Design review of the part built by this model. Coordinates are the model's own, in mm. A direction names the side the tool comes from. Give positions to 0.01 mm unless a question says otherwise; leave off trailing zeros. Write each loop counter-clockwise with the first axis right and the second up, starting at its lowest first coordinate (ties: lowest second). Pieces come first, ordered by that corner, then holes.
```python
from build123d import *

# Parameters (mm, degrees)
BOSS_EXTRUDE1_DEPTH = 304.8
SKETCH4_R           = 6.35
CUT_EXTRUDE1_DEPTH  = 599.68125614
SKETCH5_W           = 541.53125614
SKETCH5_H           = 3.114661147
BOSS_EXTRUDE2_DEPTH = 152.4


with BuildPart() as part:
    # Sketch1 → Boss-Extrude1 (new body)
    with BuildSketch(Plane(origin=(0, 0, 0), x_dir=(1, 0, 0), z_dir=(0, 1, 0))):
        Polygon((595.50625614, 4.567872613), (3.175, 4.567872613), (3.175, -53.975), (0, -53.975), (0, 0), (0, 7.742872613), (598.68125614, 7.742872613), (598.68125614, 4.567872613), (598.68125614, -49.407127387), (595.50625614, -49.407127387), align=None)
    extrude(amount=BOSS_EXTRUDE1_DEPTH)

    # Sketch4 → Cut-Extrude1 (cut, through all)
    with BuildSketch(Plane.ZY):
        with Locations((23.116063694, 152.4)):
            Circle(SKETCH4_R)
    extrude(amount=-CUT_EXTRUDE1_DEPTH, mode=Mode.SUBTRACT)

    # Sketch5 → Boss-Extrude2 (add)
    with BuildSketch(Plane(origin=(0, 304.8, 0), x_dir=(1, 0, 0), z_dir=(0, 1, 0))):
        with Locations((299.34062807, 6.088586102)):
            Rectangle(SKETCH5_W, SKETCH5_H)
    extrude(amount=BOSS_EXTRUDE2_DEPTH)


solid = part.part
```
(1) Consider section B-B, the plane z = 43. Give the boundary of the cut face in (x, y) (3 decimals).
Resolved:
outline: (0, 0) - (3.175, 0) - (3.175, 304.8) - (0, 304.8) - close; (595.506, 0) - (598.681, 0) - (598.681, 304.8) - (595.506, 304.8) - close
(2) Tool access review of faces 1 (the face through (301, 0, -7)), 2 (the face through (595.506, 150, 17)): name each direction out of +Z, -Z, +X, -X, +Y, -Y from which nothing blocks a thin tool from reaching the whole face with its end or side.
Resolved:
face 1: +Z, -Z, +X, -X, -Y
face 2: +Z, +Y, -Y
(3) Consider section D-D, the plane y = 323. Give the boundary of the cut face in (x, z) (3 decimals).
Resolved:
outline: (28.575, -7.646) - (570.106, -7.646) - (570.106, -4.531) - (28.575, -4.531) - close
(4) To check wall thickness, follow L1, parallel to X at y = 199, z = 3 (3 decimals); L2, parallel to Z at x = 1, y = 152 (3 decimals); L3, parallel to Z at x = 548, y = 109. State the ranges of each line that lie inside material, in increasing order.
Resolved:
L1: x = 0 to 3.175, 595.506 to 598.681
L2: z = -7.743 to 16.779, 29.453 to 53.975
L3: z = -7.74 to -4.57
(5) Clearance check with flat-ended pins moving along their axes: P1, Ø10, axis at x = 200, y = 339, coming from the +Z side; P2, Ø3, axis at x = 233.5, y = 206, coming from the +Z side; P3, Ø1.6, axis at y = 345, z = -6, coming from the -X side (3 decimals). State where each tip first meets the part, or that it passes through.
Resolved:
P1: stops at z = -4.53
P2: stops at z = -4.57
P3: stops at x = 28.575
(6) Mouldability with a two-part tool opening along Z and no side actions: class faces 3 (the face through (303, 150, -4.568)), 4 (the face through (598.681, 150, 15)), 5 (the face through (1.565, 158.696, 22.289)) as pulls with the +Z half, pulls with the -Z half, needs draft (parallel to the pull), parting line crosses it, or undercut.
Resolved:
face 3: pulls with the +Z half
face 4: needs draft
face 5: undercut
(7) Consider section A-A, the plane y = 152.4. Give the boundary of the cut face in (x, z) (3 decimals).
Resolved:
outline: (0, -7.743) - (598.681, -7.743) - (598.681, 16.766) - (595.506, 16.766) - (595.506, -4.568) - (3.175, -4.568) - (3.175, 16.766) - (0, 16.766) - close; (0, 29.466) - (3.175, 29.466) - (3.175, 53.975) - (0, 53.975) - close; (595.506, 29.466) - (598.681, 29.466) - (598.681, 49.407) - (595.506, 49.407) - close
